from build123d import *

# Parameters (mm, degrees)
SKETCH_1_W          = 60
SKETCH_1_H          = 50
EXTRUDE_1_DEPTH     = 10
SKETCH_2_R          = 4
CUT_EXTRUDE_1_DEPTH = 0.5
FILLET_1_R          = 3
SKETCH_3_R          = 7.5
CUT_EXTRUDE_2_DEPTH = 41.311288741


with BuildPart() as part:
    # 草图1 → 凸台-拉伸1 (new body)
    with BuildSketch(Plane(origin=(0, 0, 0), x_dir=(1, 0, 0), z_dir=(0, 1, 0))):
        Rectangle(SKETCH_1_W, SKETCH_1_H)
    extrude(amount=EXTRUDE_1_DEPTH)

    # 草图2 → 切除-拉伸1 (cut)
    with BuildSketch(Plane.XZ):
        with Locations(Location((-18, 16.9, 0), (0, 0, 270))):
            Circle(SKETCH_2_R)
        with Locations(Location((18, 16.9, 0), (0, 0, 270))):
            Circle(SKETCH_2_R)
    extrude(amount=-CUT_EXTRUDE_1_DEPTH, mode=Mode.SUBTRACT)

    # 圆角1
    fillet_1_edges = [part.edges().sort_by_distance(p)[0] for p in [
        (30, 5, 25),
        (-30, 5, 25),
    ]]
    fillet(fillet_1_edges, radius=FILLET_1_R)

    # 草图3 → 切除-拉伸2 (cut, through all)
    with BuildSketch(Plane(origin=(0, 10, 0), x_dir=(1, 0, 0), z_dir=(0, 1, 0))):
        with Locations(Location((0, -15.052922201, 0), (0, 0, 270))):
            Circle(SKETCH_3_R)
    extrude(amount=-CUT_EXTRUDE_2_DEPTH, mode=Mode.SUBTRACT)


solid = part.part
Verification items for the finished model (mm, model axes). A direction names the side the tool comes from. Coordinates: 2 decimals unless noted, no trailing zeros. Loops run counter-clockwise (first coordinate to the right, second up) from the corner with the lowest first, then second, coordinate; pieces in that order, holes last. Notation, with made-up numbers: M 44,-37 L 56,-37 A18 cw 56,-12 Z; hole C 77,60.25 d7. An arc over 180 degrees is marked long. One line per item, written item: value.
1. Section check A-A on x = 0. Record the cut outline in (y, z).
Answers follow:
outline: M 0,-25 L 10,-25 L 10,7.55 L 0,7.55 Z; M 0,22.55 L 10,22.55 L 10,25 L 0,25 Z
2. Mould release check, pull along X, two halves, no side actions. Record for faces 3 (the flat face through (-18, 0.5, 17)), 4 (the cylindrical face through (-2.87, 5.07, 21.98)), 5 (the cylindrical face through (29.1, 5.07, 24.14)), 6 (the cylindrical face through (-29.14, 5.07, 24.1)): pulls with the +X half, pulls with the -X half, needs draft (parallel to the pull), parting line crosses it, or undercut.
Answers follow:
face 3: undercut
face 4: undercut
face 5: pulls with the +X half
face 6: pulls with the -X half
3. Gauge pin test, flat ends, axial feed: P1, Ø1, axis at x = -9.5, z = 8.5, coming from the -Y side; P2, Ø6.5, axis at x = 18.5, z = 16.5, coming from the -Y side. Record the tip position at first contact, or that the pin passes through.
Answers follow:
P1: y = 0
P2: y = 0.5
4. Set-up check for faces 1 (the flat face through (30, 5, -1)), 2 (the cylindrical face through (21.373, 0.246, 14.75)): record each of +Z, -Z, +X, -X, +Y, -Y from which the full face is reachable in a straight line by a thin tool's end or side.
Answers follow:
face 1: +Z, -Z, +X, +Y, -Y
face 2: -Y
5. Section check C-C on y = 4. Record the cut outline in (x, z).
Answers follow:
outline: M -30,-25 L 30,-25 L 30,22 A3 ccw 27,25 L -27,25 A3 ccw -30,22 Z; hole C 0,15.05 d15
6. Section check B-B on z = 19. Record the cut outline in (x, y), plus the area to 3 significant figures.
Answers follow:
outline: M -30,0 L -21.4,0 L -21.4,0.5 L -14.6,0.5 L -14.6,0 L -6.38,0 L -6.38,10 L -30,10 Z; M 6.38,0 L 14.6,0 L 14.6,0.5 L 21.4,0.5 L 21.4,0 L 30,0 L 30,10 L 6.38,10 Z
area: 466 mm^2
7. Material ranges on line 1 along X through (y, z) = (0.3, 16.9); line 2 along Y through (x, z) = (-20, 13.5); line 3 along X through (y, z) = (1.25, 11.5), recorded low to high. Write a range as from..to.
Answers follow:
line 1: -30..-22, -14..-7.27, 7.27..14, 22..30
line 2: 0.5..10
line 3: -30..-6.61, 6.61..30
